```python
from build123d import *

# Parameters (mm, degrees)
F0_W     = 35.56
F0_H     = 25.4
F1_DEPTH = 3.175
F2_R     = 3.175
F2_R_2   = 1.7272
F3_DEPTH = 3.176
F4_R     = 1.5875
F5_DEPTH = 3.176


with BuildPart() as f1:
    # F0 (on Front) → F1 (new body)
    with BuildSketch(Plane.XZ):
        Rectangle(F0_W, F0_H)
    extrude(amount=F1_DEPTH)

    # F2 (on face) → F3 (cut, through all)
    with BuildSketch(Plane.XZ.offset(3.175)):
        Circle(F2_R)
        with Locations((6.604, 5.0292)):
            Circle(F2_R_2)
        with Locations((6.604, -4.318)):
            Circle(F2_R_2)
        with Locations((-6.604, -4.318)):
            Circle(F2_R_2)
        with Locations((-6.604, 5.0292)):
            Circle(F2_R_2)
    extrude(amount=-F3_DEPTH, mode=Mode.SUBTRACT)

    # F4 (on face) → F5 (cut, through all)
    with BuildSketch(Plane.XZ.offset(3.175)):
        with Locations((-13.335, 9.525)):
            Circle(F4_R)
        with Locations((13.335, -9.525)):
            Circle(F4_R)
    extrude(amount=-F5_DEPTH, mode=Mode.SUBTRACT)


solid = f1.part
```
Read the model definition and answer for the solid it produces. Units are mm, in the model's axes. Give positions to 0.01 mm unless a question says otherwise; leave off trailing zeros. Write each loop counter-clockwise with the first axis right and the second up, starting at its lowest first coordinate (ties: lowest second). Pieces come first, ordered by that corner, then holes. Notation, with made-up numbers: (8, -20) - (43, -20) arc R25 ccw to (43, 19) - close; hole circle Ø9 at (77.5, -37). An arc over 180 degrees is marked (long way). Write item = value, one per line. Start each with the question number.
Item 1: Find section D-D (z = 4.25). Give the vertices of the cut face in (x, y) (3 decimals), then the cut area to 3 significant figures.
Item 2: Find section C-C (x = 0). Give the vertices of the cut face in (y, z) (3 decimals), then the cut area to 3 significant figures.
Item 3: The mould has two halves that part along X. Classify faces 1 (the flat face through (0, -2, -12.7)), 2 (the cylindrical face through (14.85, -1.61, -9.05)), 3 (the flat face through (17.78, -2, 0)): +X half, -X half, draft (parallel to the pull), parting line (faces both ways), or undercut.
Item 4: Find section B-B (x = 6). Give the vertices of the cut face in (y, z) (3 decimals), then the cut area to 3 significant figures.
Item 5: Find the intervals of material crossed by probe 1 along X at (y, z) = (-0.9, -3.75); probe 2 along Z at (x, y) = (-6, -0.3); probe 3 along X at (y, z) = (-1.4, 5.5), in increasing order. Write a range as [from, to].
Item 6: Each of these flat-tipped pins is pushed along its axis until it touches: P1, Ø5.5, axis at x = -6.604, z = -4.318, coming from the -Y side (3 decimals); P2, Ø1.9, axis at x = -13.335, z = 9.525, coming from the +Y side (1 decimal). Where does it stop, or does it pass through?
Item 7: Find section A-A (z = 0). Give the vertices of the cut face in (x, y) (3 decimals).
Response:
q1.outline = (-17.78, -3.175) - (-8.145, -3.175) - (-8.145, 0) - (-17.78, 0) - close; (-5.063, -3.175) - (5.063, -3.175) - (5.063, 0) - (-5.063, 0) - close; (8.145, -3.175) - (17.78, -3.175) - (17.78, 0) - (8.145, 0) - close
q1.area = 93.3 mm²
q2.outline = (-3.175, -12.7) - (0, -12.7) - (0, -3.175) - (-3.175, -3.175) - close; (-3.175, 3.175) - (0, 3.175) - (0, 12.7) - (-3.175, 12.7) - close
q2.area = 60.5 mm²
q3.face_1 = draft
q3.face_2 = undercut
q3.face_3 = +X half
q4.outline = (-3.175, -12.7) - (0, -12.7) - (0, -5.936) - (-3.175, -5.936) - close; (-3.175, -2.7) - (0, -2.7) - (0, 3.411) - (-3.175, 3.411) - close; (-3.175, 6.647) - (0, 6.647) - (0, 12.7) - (-3.175, 12.7) - close
q4.area = 60.1 mm²
q5.probe_1 = [-17.78, -8.24], [-4.97, 4.97], [8.24, 17.78]
q5.probe_2 = [-12.7, -5.94], [-2.7, 3.41], [6.65, 12.7]
q5.probe_3 = [-17.78, -8.27], [-4.94, 4.94], [8.27, 17.78]
q6.P1 = -3.175
q6.P2 = through
q7.outline = (-17.78, -3.175) - (-3.175, -3.175) - (-3.175, 0) - (-17.78, 0) - close; (3.175, -3.175) - (17.78, -3.175) - (17.78, 0) - (3.175, 0) - close
